```python
from build123d import *

# Parameters (mm, degrees)
SKETCH2_R          = 1.93
CUT_EXTRUDE1_DEPTH = 27.3
CIRPATTERN1_COUNT  = 34
SKETCH6_W          = 1.65
SKETCH6_H          = 19.001
CIRPATTERN2_COUNT  = 2
CIRPATTERN2_ANGLE  = 90
SKETCH8_W          = 3.6
SKETCH8_H          = 4
CUT_EXTRUDE2_DEPTH = 29.0000001
SKETCH9_R          = 16.5
CUT_EXTRUDE3_DEPTH = 5.7


with BuildPart() as part:
    # Sketch1 → Revolve1 (revolve)
    with BuildSketch(Plane.XY):
        Polygon((-10.25, 6), (17.75, 6), (17.75, 19), (10.25, 19), (10.25, 23.5), (8.55, 23.5), (8.55, 26.485), (-8.55, 26.485), (-8.55, 23.5), (-10.25, 23.5), align=None)
    revolve(axis=Axis((0, 0, 0), (1, 0, 0)))

    # Sketch2 → Cut-Extrude1 (cut, through all)
    with BuildSketch(Plane.ZY.offset(8.55)):
        with Locations((0, 26.485)):
            Circle(SKETCH2_R)
    cut_extrude1 = extrude(amount=-CUT_EXTRUDE1_DEPTH, mode=Mode.SUBTRACT)

    # CirPattern1: Cut-Extrude1 ×34 about axis
    cirpattern1_axis = Axis((0, 0, 0), (1, 0, 0))
    for i in range(1, CIRPATTERN1_COUNT):
        add(cut_extrude1.rotate(cirpattern1_axis, i * 360 / CIRPATTERN1_COUNT), mode=Mode.SUBTRACT)

    # Sketch6 → M4x0.7 Tapped Hole1 (revolve, cut)
    with BuildSketch(Plane(origin=(14, 0, 0), x_dir=(0, 0, -1), z_dir=(1, 0, 0))):
        with Locations((0.825, 9.5005)):
            Rectangle(SKETCH6_W, SKETCH6_H)
    m4x0_7_tapped_hole1 = revolve(axis=Axis((14, -6.35, 0), (0, 1, 0)), mode=Mode.SUBTRACT)

    # CirPattern2: M4x0.7 Tapped Hole1 ×2 about axis
    cirpattern2_axis = Axis((0, 0, 0), (-1, 0, 0))
    for i in range(1, CIRPATTERN2_COUNT):
        add(m4x0_7_tapped_hole1.rotate(cirpattern2_axis, i * CIRPATTERN2_ANGLE / (CIRPATTERN2_COUNT - 1)), mode=Mode.SUBTRACT)

    # Sketch8 → Cut-Extrude2 (cut, through all)
    with BuildSketch(Plane(origin=(17.75, 0, 0), x_dir=(0, 0, -1), z_dir=(1, 0, 0))):
        with Locations((6, 0)):
            Rectangle(SKETCH8_W, SKETCH8_H)
    extrude(amount=-CUT_EXTRUDE2_DEPTH, mode=Mode.SUBTRACT)

    # Sketch9 → Cut-Extrude3 (cut)
    with BuildSketch(Plane.ZY.offset(10.25)):
        Circle(SKETCH9_R)
    extrude(amount=-CUT_EXTRUDE3_DEPTH, mode=Mode.SUBTRACT)


solid = part.part
```
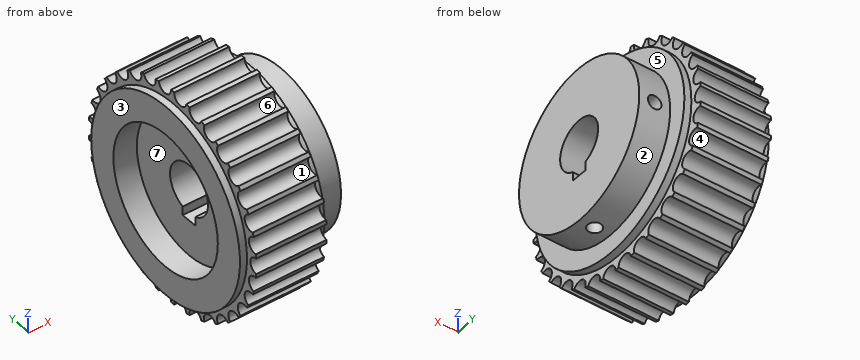
Here's how the part is built. I have some questions about the finished solid (model axes, mm). Face numbers are marked on the shaded views. A direction names the side the tool comes from. Give positions to 0.01 mm unless a question says otherwise; leave off trailing zeros. Order: outer loops, then holes, each group sorted by start corner. A loop starts at its lowest first (then second) coordinate and runs counter-clockwise, first axis right, second up. Notation, with made-up numbers: (29, -23.5) - (49, -23.5) arc R29 ccw to (49, 13.5) - close; hole circle Ø8 at (22, 70). An arc over 180 degrees is marked (long way). Answer as a JSON object with one key per item and string values. Group by question number.
Item 1: For P1, Ø4, axis at x = 13, z = 8.5, coming from the -Y side; P2, Ø2.5, axis at x = 6.5, z = -7, coming from the +Y side; P3, Ø2, axis at x = 14, y = 0, coming from the -Z side, each with a flat end and sliding along its axis, tell me the tip position at first contact or that it passes through.
Item 2: Which directions (+Z, -Z, +X, -X, +Y, -Y) give clear straight access to the entire face, cutting with the end or side of a thin tool? Please do the marked faces 5, 6 and 7.
Item 3: If we section it at D-D on y = -12.5: Please give me the cut outline in (x, z), and give its area (3 significant figures).
Item 4: Please list where these lines run through material, in increasing order: probe 1 along X at (y, z) = (0, -12.25); probe 2 along Y at (x, z) = (-7.65, 0) (3 decimals); probe 3 along Y at (x, z) = (3.75, 0) (3 decimals).
Item 5: If we section it at C-C on x = 14: Please give me the cut outline in (y, z), and give its area (3 significant figures).
Item 6: If we mould it in two halves opening along Y, with no side actions, what happens to the marked faces 1, 2, 3 and 4? For each: pulls with the +Y half, pulls with the -Y half, needs draft (parallel to the pull), parting line crosses it, or undercut.
Item 7: If we section it at A-A on z = 0: Please give me the cut outline in (x, y) (3 decimals), and give its area (3 significant figures).
Item 8: If we section it at B-B on y = 3.5: Please give me the cut outline in (x, z).
Result set:
{
 "1": {"P1": "y = -17.85", "P2": "y = 25.61", "P3": "z = 5.92"},
 "2": {"face 5": "+X", "face 6": "+X, -X", "face 7": "-X"},
 "3": {"outline": "(-10.25, -19.9) - (-8.55, -19.9) - (-8.55, -21.91) - (8.55, -21.91) - (8.55, -19.9) - (10.25, -19.9) - (10.25, -14.31) - (17.75, -14.31) - (17.75, 14.31) - (10.25, 14.31) - (10.25, 19.9) - (8.55, 19.9) - (8.55, 21.91) - (-8.55, 21.91) - (-8.55, 19.9) - (-10.25, 19.9) - (-10.25, 10.77) - (-4.55, 10.77) - (-4.55, -10.77) - (-10.25, -10.77) - close", "area": "976 mm²"},
 "4": {"probe 1": "-4.55 to 12.35, 15.65 to 17.75", "probe 2": "-24.555 to -16.5, 16.5 to 24.555", "probe 3": "-24.555 to -6, 6 to 24.555"},
 "5": {"outline": "(-2, -7.8) - (-2, -5.66) arc R6 cw (long way) to (5.77, 1.65) - (18.93, 1.65) arc R19 ccw (long way) to (-1.65, -18.93) - (-1.65, -7.8) - close; (1.65, -18.93) arc R19 ccw to (18.93, -1.65) - (5.77, -1.65) arc R6 cw to (2, -5.66) - (2, -7.8) - (1.65, -7.8) - close", "area": "933 mm²"},
 "6": {"face 1": "undercut", "face 2": "parting line crosses it", "face 3": "needs draft", "face 4": "undercut"},
 "7": {"outline": "(-10.25, -23.5) - (-8.55, -23.5) - (-8.55, -24.555) - (8.55, -24.555) - (8.55, -23.5) - (10.25, -23.5) - (10.25, -19) - (17.75, -19) - (17.75, -6) - (-4.55, -6) - (-4.55, -16.5) - (-10.25, -16.5) - close; (-10.25, 16.5) - (-4.55, 16.5) - (-4.55, 6) - (12.35, 6) - (12.35, 19) - (10.25, 19) - (10.25, 23.5) - (8.55, 23.5) - (8.55, 24.555) - (-8.55, 24.555) - (-8.55, 23.5) - (-10.25, 23.5) - close; (15.65, 6) - (17.75, 6) - (17.75, 19) - (15.65, 19) - close", "area": "786 mm²"},
 "8": {"outline": "(-10.25, -23.24) - (-8.55, -23.24) - (-8.55, -24.76) - (8.55, -24.76) - (8.55, -23.24) - (10.25, -23.24) - (10.25, -18.67) - (17.75, -18.67) - (17.75, -4.87) - (-4.55, -4.87) - (-4.55, -16.12) - (-10.25, -16.12) - close; (-10.25, 16.12) - (-4.55, 16.12) - (-4.55, 4.87) - (17.75, 4.87) - (17.75, 18.67) - (10.25, 18.67) - (10.25, 23.24) - (8.55, 23.24) - (8.55, 24.76) - (-8.55, 24.76) - (-8.55, 23.24) - (-10.25, 23.24) - close"}
}
